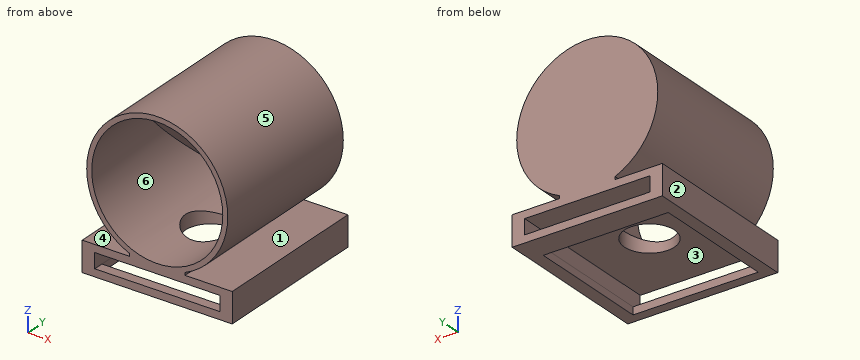
```python
from build123d import *

# Parameters (mm, degrees)
CROQUIS1_W                 = 30
CROQUIS1_H                 = 6
CROQUIS1_W_2               = 25.006000518
CROQUIS1_H_2               = 3.004001618
SALIENTE_EXTRUIR1_DEPTH    = 32.17
CROQUIS2_W                 = 25
CROQUIS2_H                 = 25.003841724
CORTAR_EXTRUIR1_DEPTH      = 1.497999
CROQUIS3_R                 = 14.098435913
CROQUIS3_R_2               = 13.1
SALIENTE_EXTRUIR2_DEPTH    = 32.17
CROQUIS10_W                = 30.177827817
CROQUIS10_H                = 41.273822818
SALIENTE_EXTRUIR4_DEPTH    = 22
CORTAR_EXTRUIR2_DEPTH      = 10
CORTAR_EXTRUIR2_DEPTH_BACK = 58
CROQUIS12_W                = 43.091208183
CROQUIS12_H                = 18.563452801
CORTAR_EXTRUIR3_DEPTH      = 58
CORTAR_EXTRUIR3_DEPTH_BACK = 58
SALIENTE_EXTRUIR6_DEPTH    = 32.17
CROQUIS22_R                = 5
CORTAR_EXTRUIR6_DEPTH      = 4


with BuildPart() as part:
    # Croquis1 → Saliente-Extruir1 (new body)
    with BuildSketch(Plane(origin=(0, 0, 0), x_dir=(1, 0, 0), z_dir=(0, 1, 0))):
        with Locations((0, 25)):
            Rectangle(CROQUIS1_W, CROQUIS1_H)
        with Locations((0, 25)):
            Rectangle(CROQUIS1_W_2, CROQUIS1_H_2, mode=Mode.SUBTRACT)
    extrude(amount=-SALIENTE_EXTRUIR1_DEPTH)

    # Croquis2 → Cortar-Extruir1 (cut)
    with BuildSketch(Plane(origin=(0, 0, -28), x_dir=(1, 0, 0), z_dir=(0, 0, -1))):
        with Locations((0, 17.668079138)):
            Rectangle(CROQUIS2_W, CROQUIS2_H)
    extrude(amount=-CORTAR_EXTRUIR1_DEPTH, mode=Mode.SUBTRACT)

    # Croquis3 → Saliente-Extruir2 (add)
    with BuildSketch(Plane(origin=(0, 0, 0), x_dir=(1, 0, 0), z_dir=(0, 1, 0))):
        with Locations((0, 8.499687815)):
            Circle(CROQUIS3_R)
        with Locations((0, 8.499687815)):
            Circle(CROQUIS3_R_2, mode=Mode.SUBTRACT)
    extrude(amount=-SALIENTE_EXTRUIR2_DEPTH)

    # Croquis10 → Saliente-Extruir4 (add)
    with BuildSketch(Plane(origin=(0, -11, -11), x_dir=(-1, 0, 0), z_dir=(0, -0.707106781, -0.707106781))):
        with Locations((-0.620676422, -5.363625683)):
            Rectangle(CROQUIS10_W, CROQUIS10_H)
    extrude(amount=-SALIENTE_EXTRUIR4_DEPTH)

    # Croquis11 → Cortar-Extruir2 (cut, two sides)
    with BuildSketch(Plane.XZ.offset(32.17)) as cortar_extruir2_sk:
        with BuildLine():
            Line((-4.676723545, -21.799843908), (-14.468237486, -21.799843908))
            Line((-14.468237486, -21.799843908), (-14.468237486, 22.941505279))
            Line((-14.468237486, 22.941505279), (15.709590331, 22.941505279))
            Line((15.709590331, 22.941505279), (15.709590331, -21.799843908))
            Line((15.709590331, -21.799843908), (4.676723545, -21.799843908))
            ThreePointArc((4.676723545, -21.799843908), (0, 5.598748098), (-4.676723545, -21.799843908))
        make_face()
    extrude(amount=CORTAR_EXTRUIR2_DEPTH, mode=Mode.SUBTRACT)
    extrude(cortar_extruir2_sk.sketch, amount=-CORTAR_EXTRUIR2_DEPTH_BACK, mode=Mode.SUBTRACT)

    # Croquis12 → Cortar-Extruir3 (cut, two sides)
    with BuildSketch(Plane(origin=(0, 0, 0), x_dir=(0, 0, -1), z_dir=(1, 0, 0))) as cortar_extruir3_sk:
        with Locations((6.454395908, 9.281726401)):
            Rectangle(CROQUIS12_W, CROQUIS12_H)
    extrude(amount=CORTAR_EXTRUIR3_DEPTH, mode=Mode.SUBTRACT)
    extrude(cortar_extruir3_sk.sketch, amount=-CORTAR_EXTRUIR3_DEPTH_BACK, mode=Mode.SUBTRACT)

    # Croquis23 → Saliente-Extruir6 (add, through all)
    with BuildSketch(Plane(origin=(0, 0, 0), x_dir=(1, 0, 0), z_dir=(0, 1, 0))):
        with BuildLine():
            Line((-5.562938112, 22), (-4.062938112, 22))
            ThreePointArc((-4.062938112, 22), (-4.820668551, 21.748350009), (-5.562938112, 21.454208831))
            Line((-5.562938112, 21.454208831), (-5.562938112, 22))
        make_face()
        with BuildLine():
            Line((4.062938112, 22), (5.562938112, 22))
            Line((5.562938112, 22), (5.562938112, 21.454208831))
            ThreePointArc((5.562938112, 21.454208831), (4.820668551, 21.748350009), (4.062938112, 22))
        make_face()
    extrude(amount=-SALIENTE_EXTRUIR6_DEPTH)

    # Croquis22 → Cortar-Extruir6 (cut)
    with BuildSketch(Plane.XY.offset(-23.497999191)):
        with Locations((0, -17.33)):
            Circle(CROQUIS22_R)
    extrude(amount=CORTAR_EXTRUIR6_DEPTH, mode=Mode.SUBTRACT)


solid = part.part
```
Verification items for the finished model (mm, model axes). Face numbers are marked on the shaded views. A direction names the side the tool comes from. Give positions to 0.01 mm unless a question says otherwise; leave off trailing zeros. Order: outer loops, then holes, each group sorted by start corner. A loop starts at its lowest first (then second) coordinate and runs counter-clockwise, first axis right, second up. Notation, with made-up numbers: M -22.5,-19 L -18.5,-19 A21 cw -18.5,8 Z; hole C -23.75,77.25 d10. An arc over 180 degrees is marked long. Answer in a Markdown table with one row per item. Add a question column.
Item 1: Section check A-A, the plane x = 0. Enter the section's corners in (y, z), and give its area (3 significant figures).
Item 2: Tool access check on the marked faces 1 and 2. Record the directions out of +Z, -Z, +X, -X, +Y, -Y that give a thin tool (end or side, any length) a straight path to the whole face; none if there is none.
Item 3: Mould release check, pull along X, two halves, no side actions. Record for the marked faces 3, 4, 5 and 6: released by +X, released by -X, zero draft, split by the parting line, or undercut.
Item 4: Gauge pin test, flat ends, axial feed: pin 1 (2 mm diameter, centred on y = -6.5, z = -2.5, fed in from -X); pin 2 (6 mm diameter, centred on y = -5, z = -3.5, fed in from +X); pin 3 (8 mm diameter, centred on y = -21.5, z = -12, fed in from +X). Record the tip position at first contact, or that the pin passes through.
Item 5: Section check C-C, the plane z = 1. Enter the section's corners in (x, y).
Item 6: Scan lines: probe 1 along Z at (x, y) = (9.5, -23.5); probe 2 along Z at (x, y) = (7.25, -30); probe 3 along X at (y, z) = (-17.33, -21.6). Record each from-to range of solid material in increasing order. Write a range as from..to.
Filled sheet:
| question | item | result |
|---|---|---|
| 1 | outline | M -32.17,-28 L -30.17,-28 L -30.17,-26.5 L -32.17,-26.5 Z; M -32.17,-23.5 L -22.33,-23.5 L -22.33,-21.6 L -32.17,-21.6 Z; M -32.17,4.6 L -26.6,4.6 L -0.4,-21.6 L -12.33,-21.6 L -12.33,-23.5 L 0,-23.5 L 0,5.6 L -32.17,5.6 Z; M -5.17,-28 L 0,-28 L 0,-26.5 L -5.17,-26.5 Z |
| 1 | area | 439 mm^2 |
| 2 | face 1 | +X, +Y, -Y |
| 2 | face 2 | +Z, -Z, -X, +Y, -Y |
| 3 | face 3 | undercut |
| 3 | face 4 | zero draft |
| 3 | face 5 | split by the parting line |
| 3 | face 6 | undercut |
| 4 | pin 1 | stops at x = -13.18 |
| 4 | pin 2 | stops at x = 13.96 |
| 4 | pin 3 | stops at x = 14.1 |
| 5 | outline | M -10.42,-32.17 L -9.02,-32.17 L -9.02,-23 L 9.02,-23 L 9.02,-32.17 L 10.42,-32.17 L 10.42,0 L -10.42,0 Z |
| 6 | probe 1 | z = -23.5..-22, -18.92..-17.52, 0.52..1.92 |
| 6 | probe 2 | z = -23.5..-22, -20.59..-19.41, 2.41..3.59 |
| 6 | probe 3 | x = -5.56..-5, 5..5.56 |
